from build123d import *

# Parameters (mm, degrees)
SKETCH_1_W          = 15
SKETCH_1_H          = 32.4
EXTRUDE_1_DEPTH     = 3
SKETCH_2_R          = 6.25
SKETCH_2_R_2        = 1.25
SKETCH_2_R_3        = 3
CUT_EXTRUDE_1_DEPTH = 124.493967464
SKETCH_2_3_R        = 2
CUT_EXTRUDE_2_DEPTH = 1.5
SKETCH_4_R          = 0.8
CUT_EXTRUDE_3_DEPTH = 124.493967464
SKETCH_5_R          = 0.8
CUT_EXTRUDE_4_DEPTH = 3


with BuildPart() as part:
    # Sketch 1 → Extrude 1 (new body)
    with BuildSketch(Plane(origin=(0, 0, 0), x_dir=(1, 0, 0), z_dir=(0, 1, 0))):
        with Locations((7.5, 16.2)):
            Rectangle(SKETCH_1_W, SKETCH_1_H)
        Polygon((15, 0), (0, 0), (0, -40), (15, -40), (85, -40), (100, -40), (100, 0), (85, 0), align=None)
        with Locations((7.5, -56.2)):
            Rectangle(SKETCH_1_W, SKETCH_1_H)
        with Locations((92.5, 16.2)):
            Rectangle(SKETCH_1_W, SKETCH_1_H)
        with Locations((92.5, -56.2)):
            Rectangle(SKETCH_1_W, SKETCH_1_H)
    extrude(amount=EXTRUDE_1_DEPTH)

    # Sketch 2 → Cut-Extrude 1 (cut, through all)
    with BuildSketch(Plane.XZ):
        with Locations((7.5, -21.35)):
            Circle(SKETCH_2_R)
        with Locations(Location((3, -3, 0), (0, 0, 270))):
            Circle(SKETCH_2_R_2)
        with Locations(Location((12, -3, 0), (0, 0, 270))):
            Circle(SKETCH_2_R_2)
        with Locations(Location((12, -29.4, 0), (0, 0, 270))):
            Circle(SKETCH_2_R_2)
        with Locations(Location((3, -29.4, 0), (0, 0, 270))):
            Circle(SKETCH_2_R_2)
        with Locations((7.5, -15.6)):
            Circle(SKETCH_2_R_3)
        with Locations((92.5, -21.35)):
            Circle(SKETCH_2_R)
        with Locations((92.5, -15.6)):
            Circle(SKETCH_2_R_3)
        with Locations(Location((88, -3, 0), (0, 0, 270))):
            Circle(SKETCH_2_R_2)
        with Locations(Location((97, -3, 0), (0, 0, 270))):
            Circle(SKETCH_2_R_2)
        with Locations(Location((88, -29.4, 0), (0, 0, 270))):
            Circle(SKETCH_2_R_2)
        with Locations(Location((97, -29.4, 0), (0, 0, 270))):
            Circle(SKETCH_2_R_2)
        with Locations((92.5, 61.35)):
            Circle(SKETCH_2_R)
        with Locations((92.5, 55.6)):
            Circle(SKETCH_2_R_3)
        with Locations(Location((88, 69.4, 0), (0, 0, 270))):
            Circle(SKETCH_2_R_2)
        with Locations(Location((97, 69.4, 0), (0, 0, 270))):
            Circle(SKETCH_2_R_2)
        with Locations(Location((88, 43, 0), (0, 0, 270))):
            Circle(SKETCH_2_R_2)
        with Locations(Location((97, 43, 0), (0, 0, 270))):
            Circle(SKETCH_2_R_2)
        with Locations(Location((3, 69.4, 0), (0, 0, 270))):
            Circle(SKETCH_2_R_2)
        with Locations(Location((12, 69.4, 0), (0, 0, 270))):
            Circle(SKETCH_2_R_2)
        with Locations((7.5, 61.35)):
            Circle(SKETCH_2_R)
        with Locations((7.5, 55.6)):
            Circle(SKETCH_2_R_3)
        with Locations(Location((3, 43, 0), (0, 0, 270))):
            Circle(SKETCH_2_R_2)
        with Locations(Location((12, 43, 0), (0, 0, 270))):
            Circle(SKETCH_2_R_2)
    extrude(amount=-CUT_EXTRUDE_1_DEPTH, mode=Mode.SUBTRACT)

    # Sketch 2_3 → Cut-Extrude 2 (cut)
    with BuildSketch(Plane.XZ):
        with Locations(Location((3, -29.4, 0), (0, 0, 270))):
            Circle(SKETCH_2_3_R)
        with Locations(Location((3, -3, 0), (0, 0, 270))):
            Circle(SKETCH_2_3_R)
        with Locations(Location((12, -3, 0), (0, 0, 270))):
            Circle(SKETCH_2_3_R)
        with Locations(Location((12, -29.4, 0), (0, 0, 270))):
            Circle(SKETCH_2_3_R)
        with Locations(Location((88, -3, 0), (0, 0, 270))):
            Circle(SKETCH_2_3_R)
        with Locations(Location((97, -3, 0), (0, 0, 270))):
            Circle(SKETCH_2_3_R)
        with Locations(Location((88, -29.4, 0), (0, 0, 270))):
            Circle(SKETCH_2_3_R)
        with Locations(Location((97, -29.4, 0), (0, 0, 270))):
            Circle(SKETCH_2_3_R)
        with Locations(Location((88, 69.4, 0), (0, 0, 270))):
            Circle(SKETCH_2_3_R)
        with Locations(Location((97, 69.4, 0), (0, 0, 270))):
            Circle(SKETCH_2_3_R)
        with Locations(Location((88, 43, 0), (0, 0, 270))):
            Circle(SKETCH_2_3_R)
        with Locations(Location((97, 43, 0), (0, 0, 270))):
            Circle(SKETCH_2_3_R)
        with Locations(Location((3, 69.4, 0), (0, 0, 270))):
            Circle(SKETCH_2_3_R)
        with Locations(Location((12, 69.4, 0), (0, 0, 270))):
            Circle(SKETCH_2_3_R)
        with Locations(Location((3, 43, 0), (0, 0, 270))):
            Circle(SKETCH_2_3_R)
        with Locations(Location((12, 43, 0), (0, 0, 270))):
            Circle(SKETCH_2_3_R)
    extrude(amount=-CUT_EXTRUDE_2_DEPTH, mode=Mode.SUBTRACT)

    # Sketch 4 → Cut-Extrude 3 (cut, through all)
    with BuildSketch(Plane(origin=(0, 3, 0), x_dir=(1, 0, 0), z_dir=(0, 1, 0))):
        with Locations(Location((3, -4, 0), (0, 0, 270))):
            Circle(SKETCH_4_R)
        with Locations(Location((3, -36, 0), (0, 0, 270))):
            Circle(SKETCH_4_R)
        with Locations(Location((97, -36, 0), (0, 0, 270))):
            Circle(SKETCH_4_R)
        with Locations(Location((97, -4, 0), (0, 0, 270))):
            Circle(SKETCH_4_R)
    extrude(amount=-CUT_EXTRUDE_3_DEPTH, mode=Mode.SUBTRACT)

    # Sketch 5 → Cut-Extrude 4 (cut)
    with BuildSketch(Plane(origin=(0, 3, 0), x_dir=(1, 0, 0), z_dir=(0, 1, 0))):
        with Locations(Location((14.75, -5, 0), (0, 0, 270))):
            Circle(SKETCH_5_R)
        with Locations(Location((24.75, -5, 0), (0, 0, 270))):
            Circle(SKETCH_5_R)
        with Locations(Location((34.75, -5, 0), (0, 0, 270))):
            Circle(SKETCH_5_R)
        with Locations(Location((44.75, -5, 0), (0, 0, 270))):
            Circle(SKETCH_5_R)
        with Locations(Location((54.75, -5, 0), (0, 0, 270))):
            Circle(SKETCH_5_R)
        with Locations(Location((64.75, -5, 0), (0, 0, 270))):
            Circle(SKETCH_5_R)
        with Locations(Location((74.75, -5, 0), (0, 0, 270))):
            Circle(SKETCH_5_R)
        with Locations(Location((84.75, -5, 0), (0, 0, 270))):
            Circle(SKETCH_5_R)
        with Locations(Location((24.75, -15, 0), (0, 0, 270))):
            Circle(SKETCH_5_R)
        with Locations(Location((34.75, -15, 0), (0, 0, 270))):
            Circle(SKETCH_5_R)
        with Locations(Location((44.75, -15, 0), (0, 0, 270))):
            Circle(SKETCH_5_R)
        with Locations(Location((54.75, -15, 0), (0, 0, 270))):
            Circle(SKETCH_5_R)
        with Locations(Location((64.75, -15, 0), (0, 0, 270))):
            Circle(SKETCH_5_R)
        with Locations(Location((74.75, -15, 0), (0, 0, 270))):
            Circle(SKETCH_5_R)
        with Locations(Location((84.75, -15, 0), (0, 0, 270))):
            Circle(SKETCH_5_R)
        with Locations(Location((24.75, -25, 0), (0, 0, 270))):
            Circle(SKETCH_5_R)
        with Locations(Location((34.75, -25, 0), (0, 0, 270))):
            Circle(SKETCH_5_R)
        with Locations(Location((44.75, -25, 0), (0, 0, 270))):
            Circle(SKETCH_5_R)
        with Locations(Location((54.75, -25, 0), (0, 0, 270))):
            Circle(SKETCH_5_R)
        with Locations(Location((64.75, -25, 0), (0, 0, 270))):
            Circle(SKETCH_5_R)
        with Locations(Location((74.75, -25, 0), (0, 0, 270))):
            Circle(SKETCH_5_R)
        with Locations(Location((84.75, -25, 0), (0, 0, 270))):
            Circle(SKETCH_5_R)
        with Locations(Location((24.75, -35, 0), (0, 0, 270))):
            Circle(SKETCH_5_R)
        with Locations(Location((34.75, -35, 0), (0, 0, 270))):
            Circle(SKETCH_5_R)
        with Locations(Location((44.75, -35, 0), (0, 0, 270))):
            Circle(SKETCH_5_R)
        with Locations(Location((54.75, -35, 0), (0, 0, 270))):
            Circle(SKETCH_5_R)
        with Locations(Location((64.75, -35, 0), (0, 0, 270))):
            Circle(SKETCH_5_R)
        with Locations(Location((74.75, -35, 0), (0, 0, 270))):
            Circle(SKETCH_5_R)
        with Locations(Location((84.75, -35, 0), (0, 0, 270))):
            Circle(SKETCH_5_R)
        with Locations(Location((14.75, -15, 0), (0, 0, 270))):
            Circle(SKETCH_5_R)
        with Locations(Location((14.75, -25, 0), (0, 0, 270))):
            Circle(SKETCH_5_R)
        with Locations(Location((14.75, -35, 0), (0, 0, 270))):
            Circle(SKETCH_5_R)
    extrude(amount=-CUT_EXTRUDE_4_DEPTH, mode=Mode.SUBTRACT)


solid = part.part
The model under review builds one solid part; all positions refer to its coordinate system, in mm. A direction names the side the tool comes from. Give positions to 0.01 mm unless a question says otherwise; leave off trailing zeros. Loops run counter-clockwise (first coordinate to the right, second up) from the corner with the lowest first, then second, coordinate; pieces in that order, holes last. Notation, with made-up numbers: (89, 2.25) -> (130, 2.25) arc R18 ccw to (130, 11.25) -> close; hole circle Ø7 at (43, 70.5). An arc over 180 degrees is marked (long way). Put each result on its own line as item: value. Start each with the question number.
1. We need section A-A on z = -21.35. State the section outline as (x, y) points.
2. Mouldability with a two-part tool opening along Z and no side actions: class faces 4 (the face through (85, 1, 56)), 5 (the face through (12.088, 0.74, -27.402)), 6 (the face through (92, 1, -32.4)), 7 (the face through (2.521, 2.24, -30.555)) as released by +Z, released by -Z, zero draft, split by the parting line, or undercut.
3. We need section B-B on z = -3. State how many separate pieces and enclosed holes the cut face has, then the cut area to 3 significant figures.
4. Wall thickness on probe 1 along X at (y, z) = (0.2, 55.5); probe 2 along Z at (x, y) = (64.75, 2); probe 3 along X at (y, z) = (1.2, -3): over which ranges is each line inside the solid? List them lowest first.
5. Clearance check with a flat-ended pin moving along its axis: P1, Ø2, axis at x = 88, z = -28.5, coming from the -Y side. State where the tip first meets the part, or that it passes through.
6. We need section C-C on x = 30. State the section outline as (y, z) points.
7. For faces 1 (the face through (98.983, 0.74, -29.14)), 2 (the face through (3.38, 2.24, -4.19)), 3 (the face through (85, 1, -16)), list the 3-axis set-ups (+Z, -Z, +X, -X, +Y, -Y) from which the entire face can be reached by the end or side of a thin tool; tool diameter is ignored.
Determined:
1. outline: (0, 0) -> (1.25, 0) -> (1.25, 3) -> (0, 3) -> close; (13.75, 0) -> (15, 0) -> (15, 3) -> (13.75, 3) -> close; (85, 0) -> (86.25, 0) -> (86.25, 3) -> (85, 3) -> close; (98.75, 0) -> (100, 0) -> (100, 3) -> (98.75, 3) -> close
2. face 4: zero draft
2. face 5: undercut
2. face 6: released by -Z
2. face 7: undercut
3. separate pieces: 6
3. enclosed holes: 0
3. area: 51.0 mm^2
4. probe 1: 0 to 4.5, 10.5 to 15, 85 to 89.5, 95.5 to 100
4. probe 2: 0 to 4.2, 5.8 to 14.2, 15.8 to 24.2, 25.8 to 34.2, 35.8 to 40
4. probe 3: 0 to 1, 5 to 10, 14 to 15, 85 to 86, 90 to 95, 99 to 100
5. P1: y = 1.5
6. outline: (0, 0) -> (3, 0) -> (3, 40) -> (0, 40) -> close
7. face 1: -Y
7. face 2: +Y, -Y
7. face 3: -Z, +Y, -Y
